```python
from build123d import *

# Parameters (mm, degrees)
F0_W     = 7.2151930332
F0_H     = 6.6723177403
F1_DEPTH = 9.55
F2_DEPTH = 7.55
F3_DEPTH = 1


with BuildPart() as f1:
    # F0 (on Top) → F1 (new body)
    with BuildSketch(Plane.XY):
        Polygon((-80.6037993431, 76.7011865973), (-80.6037993431, 83.3735043377), (-83.6037993431, 83.3735043377), (-83.6037993431, -11.0764956623), (77.3962006569, -11.0764956623), (77.3962006569, 83.3735043377), (74.3962006569, 83.3735043377), (74.3962006569, 76.7011865973), (74.3962006569, 7.9235043377), (74.3962006569, -8.0764956623), (61.3962006569, -8.0764956623), (-67.6037993431, -8.0764956623), (-80.6037993431, -8.0764956623), (-80.6037993431, 7.9235043377), align=None)
        Polygon((-67.6037993431, -8.0764956623), (-80.6037993431, 7.9235043377), (-80.6037993431, -8.0764956623), align=None)
        Polygon((74.3962006569, 7.9235043377), (61.3962006569, -8.0764956623), (74.3962006569, -8.0764956623), align=None)
        Polygon((67.1810076237, 83.3735043377), (-73.3886063099, 83.3735043377), (-73.3886063099, 76.7011865973), (-80.6037993431, 76.7011865973), (-80.6037993431, 7.9235043377), (-67.6037993431, -8.0764956623), (61.3962006569, -8.0764956623), (74.3962006569, 7.9235043377), (74.3962006569, 76.7011865973), (67.1810076237, 76.7011865973), align=None)
        with Locations((70.7886041403, 80.0373454675)):
            Rectangle(F0_W, F0_H)
        with Locations((-76.9962028265, 80.0373454675)):
            Rectangle(F0_W, F0_H)
    extrude(amount=F1_DEPTH)

    # F0 (on Top) → F2 (cut)
    with BuildSketch(Plane.XY):
        Polygon((67.1810076237, 83.3735043377), (-73.3886063099, 83.3735043377), (-73.3886063099, 76.7011865973), (-80.6037993431, 76.7011865973), (-80.6037993431, 7.9235043377), (-67.6037993431, -8.0764956623), (61.3962006569, -8.0764956623), (74.3962006569, 7.9235043377), (74.3962006569, 76.7011865973), (67.1810076237, 76.7011865973), align=None)
        Polygon((-67.6037993431, -8.0764956623), (-80.6037993431, 7.9235043377), (-80.6037993431, -8.0764956623), align=None)
        Polygon((74.3962006569, 7.9235043377), (61.3962006569, -8.0764956623), (74.3962006569, -8.0764956623), align=None)
        with Locations((70.7886041403, 80.0373454675)):
            Rectangle(F0_W, F0_H)
        with Locations((-76.9962028265, 80.0373454675)):
            Rectangle(F0_W, F0_H)
    extrude(amount=F2_DEPTH, mode=Mode.SUBTRACT)

    # F0 (on Top) → F3 (join)
    with BuildSketch(Plane.XY):
        Polygon((-67.6037993431, -8.0764956623), (-80.6037993431, 7.9235043377), (-80.6037993431, -8.0764956623), align=None)
        Polygon((74.3962006569, 7.9235043377), (61.3962006569, -8.0764956623), (74.3962006569, -8.0764956623), align=None)
        with Locations((70.7886041403, 80.0373454675)):
            Rectangle(F0_W, F0_H)
        with Locations((-76.9962028265, 80.0373454675)):
            Rectangle(F0_W, F0_H)
    extrude(amount=F3_DEPTH)


solid = f1.part
```
Source: CAD feature listing. Evaluate the final solid. Frame: model axes, mm. A direction names the side the tool comes from. Coordinates: 2 decimals unless noted, no trailing zeros. Loops run counter-clockwise (first coordinate to the right, second up) from the corner with the lowest first, then second, coordinate; pieces in that order, holes last. Notation, with made-up numbers: M -12,-13 L 22,-13 A24 ccw 22,16 Z; hole C 27,-14.75 d2. An arc over 180 degrees is marked long. Use a Markdown table: item, result. Add a question column.
Q1. Draft query along X for faces 4 (the flat face through (-80.604, 38, 4)), 5 (the flat face through (-83.604, 37, 5)), 6 (the flat face through (-4, -11.076, 5)). Return one class per face: pulls with the +X half, pulls with the -X half, needs draft (parallel to the pull), parting line crosses it, or undercut.
Q2. Section query A-A, the plane y = 44. Return loops of the section in (x, z), and give its area (3 significant figures).
Q3. Section query C-C, the plane x = -8. Return loops of the section in (y, z), and give its area (3 significant figures).
Q4. Access query for faces 1 (the flat face through (3, 83.374, 8)), 2 (the flat face through (-77, -4, 1)), 3 (the flat face through (-74.01, -0.19, 0.49)). Directions: +Z, -Z, +X, -X, +Y, -Y. A direction counts if a zero-diameter tool reaches every point of the face in a straight line with its end or side. Return the directions, or none.
Q5. Section query B-B, the plane z = 4. Return loops of the section in (x, y).
Q6. Material intervals for L1, parallel to X at y = 3, z = 3.75; L2, parallel to Y at x = 11.5, z = 3.75; L3, parallel to Z at x = 29.5, y = 12.5, sorted ascending.
Q7. First-contact query: pin 1 (4 mm diameter, centred on x = -11.5, z = 2, fed in from +Y); pin 2 (10 mm diameter, centred on x = -62, y = 6, fed in from -Z). Flat tips, straight axial feed; report the tip coordinate or a pass-through.
Result:
| question | item | result |
|---|---|---|
| 1 | face 4 | undercut |
| 1 | face 5 | pulls with the -X half |
| 1 | face 6 | needs draft |
| 2 | outline | M -83.6,0 L -80.6,0 L -80.6,7.55 L 74.4,7.55 L 74.4,0 L 77.4,0 L 77.4,9.55 L -83.6,9.55 Z |
| 2 | area | 367 mm2 |
| 3 | outline | M -11.08,0 L -8.08,0 L -8.08,7.55 L 83.37,7.55 L 83.37,9.55 L -11.08,9.55 Z |
| 3 | area | 212 mm2 |
| 4 | face 1 | +Z, -Z, +X, -X, +Y |
| 4 | face 2 | +Y |
| 4 | face 3 | -Z |
| 5 | outline | M -83.6,-11.08 L 77.4,-11.08 L 77.4,83.37 L 74.4,83.37 L 74.4,-8.08 L -80.6,-8.08 L -80.6,83.37 L -83.6,83.37 Z |
| 6 | L1 | x = -83.6 to -80.6, 74.4 to 77.4 |
| 6 | L2 | y = -11.08 to -8.08 |
| 6 | L3 | z = 7.55 to 9.55 |
| 7 | pin 1 | stops at y = -8.08 |
| 7 | pin 2 | stops at z = 7.55 |
